from build123d import *

# Parameters (mm, degrees)
F0_W     = 22.3
F0_H     = 22
F1_DEPTH = 15
F3_START = 15
F2_R     = 7.5
F3_DEPTH = 12
F5_START = -9
F4_R     = 1
F5_DEPTH = 3
F6_START = 9
F6_DEPTH = 4


with BuildPart() as f1:
    # F0 (on Top) → F1 (new body)
    with BuildSketch(Plane.XY):
        Rectangle(F0_W, F0_H)
    extrude(amount=F1_DEPTH)

    # F2 (on Top) → F3 (join)
    with BuildSketch(Plane.XY.offset(F3_START)):
        Circle(F2_R)
    extrude(amount=F3_DEPTH)

    # F4 (on Right) → F5 (cut)
    with BuildSketch(Plane.YZ.offset(F5_START)):
        with Locations((6, 12.4410456046)):
            Circle(F4_R)
        with Locations((0, 12.4410456046)):
            Circle(F4_R)
        with Locations((-6, 12.4410456046)):
            Circle(F4_R)
    extrude(amount=-F5_DEPTH, mode=Mode.SUBTRACT)

    # F4 (on Right) → F6 (cut)
    with BuildSketch(Plane.YZ.offset(F6_START)):
        with Locations((6, 12.4410456046)):
            Circle(F4_R)
        with Locations((0, 12.4410456046)):
            Circle(F4_R)
        with Locations((-6, 12.4410456046)):
            Circle(F4_R)
    extrude(amount=F6_DEPTH, mode=Mode.SUBTRACT)


solid = f1.part
Model file for the job. Use its own axes, mm. A direction names the side the tool comes from. Give positions to 0.01 mm unless a question says otherwise; leave off trailing zeros. Order: outer loops, then holes, each group sorted by start corner. A loop starts at its lowest first (then second) coordinate and runs counter-clockwise, first axis right, second up. Notation, with made-up numbers: (-16, 74) - (1, 74) arc R16 ccw to (1, 79) - close; hole circle Ø9 at (74.25, 87). An arc over 180 degrees is marked (long way). One line per item, written item: value.
Item 1: Tool access for faces 4 (the cylindrical face through (-7.493, 0.33, 20.916)), 5 (the flat face through (-9, -6, 12)), 6 (the cylindrical face through (10.06, 5.21, 11.83)): list every direction of +Z, -Z, +X, -X, +Y, -Y with a clear straight run to the whole face (end or side of a thin tool).
Response values:
face 4: +Z
face 5: -X
face 6: +X
Item 2: Slice it at B-B (x = 0). List the corners of the cut face in (y, z), then the cut area to 3 significant figures.
Response values:
outline: (-11, 0) - (11, 0) - (11, 15) - (7.5, 15) - (7.5, 27) - (-7.5, 27) - (-7.5, 15) - (-11, 15) - close
area: 510 mm2
Item 3: Pin check, flat tips, straight feed: pin 1 Ø2.5 at (y, z) = (6, 12.44) entering from -X; pin 2 Ø3 at (x, z) = (-5, 21) entering from +Y; pin 3 Ø1.8 at (y, z) = (-6, 12.44) entering from +X; pin 4 Ø1.2 at (y, z) = (-6, 12.44) entering from -X. Stop position of each tip, or through.
Response values:
pin 1: x = -11.15
pin 2: y = 6.63
pin 3: x = 9
pin 4: x = -9
Item 4: Slice it at A-A (y = 0). List the corners of the cut face in (x, z).
Response values:
outline: (-11.15, 0) - (11.15, 0) - (11.15, 11.44) - (9, 11.44) - (9, 13.44) - (11.15, 13.44) - (11.15, 15) - (7.5, 15) - (7.5, 27) - (-7.5, 27) - (-7.5, 15) - (-11.15, 15) - (-11.15, 13.44) - (-9, 13.44) - (-9, 11.44) - (-11.15, 11.44) - close
Item 5: Slice it at C-C (z = 18.5). List the corners of the cut face in (x, y).
Response values:
outline: circle Ø15 at (0, 0)
Item 6: Two-plate mould, pull along Y, no slides. Class faces 1 (the flat face through (9, 6, 12)), 2 (the flat face through (11.15, 0, 7)), 3 (the flat face through (0, -11, 7)): released by +Y, released by -Y, zero draft, split by the parting line, or undercut.
Response values:
face 1: undercut
face 2: zero draft
face 3: released by -Y
Item 7: Wall check: line 1 (Z direction, x = -10.35, y = 6); line 2 (Z direction, x = 8.25, y = -0.5); line 3 (Y direction, x = 0.25, z = 19.5). Give the ranges that are in metal, low to high.
Response values:
line 1: 0 to 11.44, 13.44 to 15
line 2: 0 to 15
line 3: -7.5 to 7.5
Item 8: Slice it at D-D (y = -6). List the corners of the cut face in (x, z).
Response values:
outline: (-11.15, 0) - (11.15, 0) - (11.15, 11.44) - (9, 11.44) - (9, 13.44) - (11.15, 13.44) - (11.15, 15) - (4.5, 15) - (4.5, 27) - (-4.5, 27) - (-4.5, 15) - (-11.15, 15) - (-11.15, 13.44) - (-9, 13.44) - (-9, 11.44) - (-11.15, 11.44) - close
